Source: CAD feature listing. Evaluate the final solid. Frame: model axes, mm. A direction names the side the tool comes from. Coordinates: 2 decimals unless noted, no trailing zeros. Loops run counter-clockwise (first coordinate to the right, second up) from the corner with the lowest first, then second, coordinate; pieces in that order, holes last.
Item 1: Pull-direction query (X, two-part tool) for faces 1 (the cylindrical face through (-2.919, 3.072, 1.204)), 2 (the cylindrical face through (-2.32, -10.446, 3.423)), 3 (the flat face through (0, 0, 9)); classes: +X half, -X half, draft (parallel to the pull), parting line (faces both ways), or undercut.
Item 2: Section query B-B, the plane y = 0. Return the cut outline in (x, z), then the cut area to 4 significant figures.
Item 3: Section query A-A, the plane z = 2.25. Return the cut outline in (x, y) (3 decimals), then the cut area to 3 significant figures.
Item 4: Line query: probe 1 along Y at (x, z) = (0, 2.25); probe 2 along X at (y, z) = (1, 4.75); probe 3 along X at (y, z) = (-0.75, 3.5). Output: solid intervals per line, ascending.
Item 5: Pin query (flat end, axial travel): pin 1 Ø5 at (y, z) = (3, 0.5) entering from -X; pin 2 Ø1.5 at (x, z) = (-2.5, 2) entering from -Y; pin 3 Ø5 at (x, z) = (4.5, 0.5) entering from -Y. Return the tip coordinate at first contact, or that it passes through.
Item 6: Reachability of faces 4 (the flat face through (-2, 4, -2)), 5 (the cylindrical face through (3.25, 0.04, 1.2)) from +Z, -Z, +X, -X, +Y, -Y: full face, straight path, thin tool, end or side. Return the list, or none.
Item 7: Section query D-D, the plane x = 4.25. Return the cut outline in (y, z), then the cut area to 3 significant figures.
Item 8: Section query C-C, the plane x = -6. Return the cut outline in (y, z), then the cut area to 3 significant figures.
```python
from build123d import *

# Parameters (mm, degrees)
CYLINDER157_R     = 2.25
CYLINDER157_DEPTH = 7
CYLINDER156_R     = 1
CYLINDER156_DEPTH = 14
CYLINDER147_R     = 1
CYLINDER147_DEPTH = 1
ARRAY_COUNT       = 3
CYLINDER153_R     = 10
CYLINDER153_DEPTH = 10
CYLINDER_R        = 10.7
CYLINDER_DEPTH    = 11


with BuildPart() as sealsubtraction:
    # Cylinder157 → Cylinder157 (new body)
    with BuildSketch(Plane.XY.offset(4.5)):
        Circle(CYLINDER157_R)
    extrude(amount=CYLINDER157_DEPTH)


with BuildPart() as bottomwireoutlet:
    # Cylinder156 → Cylinder156 (new body)
    with BuildSketch(Plane.XY.offset(-7)):
        Circle(CYLINDER156_R)
    extrude(amount=CYLINDER156_DEPTH)


with BuildPart() as sealarray:
    # Cylinder147 → Cylinder147 (new body)
    with BuildSketch(Plane.XY.offset(4.5)):
        Circle(CYLINDER147_R)
    extrude(amount=CYLINDER147_DEPTH)

    # Fusion: union SealSubtraction, BottomWireOutlet
    add(sealsubtraction.part)
    add(bottomwireoutlet.part)


with BuildPart() as sealarray_1:
    # Fusion placement: moved
    add(sealarray.part.moved(Location((4.25, 0, 0))))

    # Array: SealArray ×3 about axis
    array_axis = Axis((0, 0, 0), (0, 0, 1))


with BuildPart() as sealarray_2:
    add(sealarray_1.part)
    for i in range(1, ARRAY_COUNT):
        add(sealarray_1.part.rotate(array_axis, i * 360 / ARRAY_COUNT))


with BuildPart() as cut:
    # Cylinder153 → Cylinder153 (new body)
    with BuildSketch(Plane.XY.offset(-2)):
        Circle(CYLINDER153_R)
    extrude(amount=CYLINDER153_DEPTH)

    # Cut: cut SealArray
    add(sealarray_2.part, mode=Mode.SUBTRACT)


with BuildPart() as cut027:
    # Cylinder → Cylinder (new body)
    with BuildSketch(Plane.XY.offset(-2)):
        Circle(CYLINDER_R)
    extrude(amount=CYLINDER_DEPTH)

    # Cut027: cut Cut
    add(cut.part, mode=Mode.SUBTRACT)


solid = cut027.part
```
Verdict:
1. face 1: undercut
1. face 2: parting line
1. face 3: draft
2. outline: (-10.7, -2) - (-10, -2) - (-10, 8) - (2, 8) - (2, 4.5) - (3.25, 4.5) - (3.25, -2) - (5.25, -2) - (5.25, 4.5) - (6.5, 4.5) - (6.5, 8) - (10, 8) - (10, -2) - (10.7, -2) - (10.7, 9) - (-10.7, 9) - close
2. area: 64.15 mm2
3. outline: circle Ø21.4 at (0, 0); circle Ø2 at (-2.125, -3.681); circle Ø2 at (-2.125, 3.681); circle Ø2 at (4.25, 0); hole circle Ø20 at (0, 0)
3. area: 54.9 mm2
4. probe 1: y = -10.7 to -10, 10 to 10.7
4. probe 2: x = -10.65 to -9.95, 2.23 to 6.27, 9.95 to 10.65
4. probe 3: x = -10.67 to -9.97, 3.59 to 4.91, 9.97 to 10.67
5. pin 1: stops at x = -10.69
5. pin 2: stops at y = -10.56
5. pin 3: stops at y = -10.51
6. face 4: -Z, +X, -X, +Y, -Y
6. face 5: -Z
7. outline: (-9.82, -2) - (-9.05, -2) - (-9.05, 8) - (-2.25, 8) - (-2.25, 4.5) - (-1, 4.5) - (-1, -2) - (1, -2) - (1, 4.5) - (2.25, 4.5) - (2.25, 8) - (9.05, 8) - (9.05, -2) - (9.82, -2) - (9.82, 9) - (-9.82, 9) - close
7. area: 63.7 mm2
8. outline: (-8.86, -2) - (-8, -2) - (-8, 8) - (8, 8) - (8, -2) - (8.86, -2) - (8.86, 9) - (-8.86, 9) - close
8. area: 34.9 mm2
